```python
from build123d import *

# Parameters (mm, degrees)
SKETCH1_W           = 37
SKETCH1_H           = 22.3
BOSS_EXTRUDE1_DEPTH = 19.13
BOSS_EXTRUDE2_DEPTH = 22.3


with BuildPart() as part:
    # Sketch1 → Boss-Extrude1 (new body)
    with BuildSketch(Plane(origin=(0, 0, 0), x_dir=(1, 0, 0), z_dir=(0, 1, 0))):
        Rectangle(SKETCH1_W, SKETCH1_H)
    extrude(amount=BOSS_EXTRUDE1_DEPTH)

    # Sketch2 → Boss-Extrude2 (add)
    with BuildSketch(Plane.XY.offset(11.15)):
        with BuildLine():
            Line((4e-09, 0), (-18.5, 0))
            Line((-18.5, 0), (-18.5, -18.5))
            ThreePointArc((-18.5, -18.5), (-13.081475451, -5.418524547), (4e-09, 0))
        make_face()
        with BuildLine():
            Line((18.5, 0), (4e-09, 0))
            ThreePointArc((4e-09, 0), (13.081475453, -5.418524549), (18.5, -18.5))
            Line((18.5, -18.5), (18.5, 0))
        make_face()
    extrude(amount=-BOSS_EXTRUDE2_DEPTH)


solid = part.part
```
Verification items for the finished model (mm, model axes). Round coordinates to 2 decimals unless told otherwise and drop trailing zeros. Order: outer loops, then holes, each group sorted by start corner. A loop starts at its lowest first (then second) coordinate and runs counter-clockwise, first axis right, second up. Notation, with made-up numbers: (-29.75, -6) -> (15.25, -6) arc R27 cw to (15.25, 23) -> close; hole circle Ø3 at (36.5, 40.25). An arc over 180 degrees is marked (long way). Put each result on its own line as item: value. Start each with the question number.
(1) Section check A-A (y = -9). Enter the section's corners in (x, z), then the cut area to 3 significant figures.
(2) Depth check by flat-ended pin: pin 1 Ø3 at (x, z) = (-9, 4) entering from -Y; pin 2 Ø10 at (x, y) = (5.5, -8.5) entering from -Z. Enter the tip coordinate at first touch or a pass-through.
(3) Material ranges on line 1 along X through (y, z) = (-15, 0); line 2 along X through (y, z) = (-4, 0); line 3 along Y through (x, z) = (-2.5, 0), recorded low to high.
(4) Section check B-B (z = -7.25). Enter the section's corners in (x, y).
(5) Section check C-C (x = 6). Enter the section's corners in (y, z).
Completed:
1. outline: (-18.5, -11.15) -> (-15.87, -11.15) -> (-15.87, 11.15) -> (-18.5, 11.15) -> close; (15.87, -11.15) -> (18.5, -11.15) -> (18.5, 11.15) -> (15.87, 11.15) -> close
1. area: 117 mm2
2. pin 1: stops at y = -3.27
2. pin 2: passes through
3. line 1: x = -18.5 to -18.17, 18.17 to 18.5
3. line 2: x = -18.5 to -11.49, 11.49 to 18.5
3. line 3: y = -0.17 to 19.13
4. outline: (-18.5, -18.5) arc R18.5 cw to (18.5, -18.5) -> (18.5, 19.13) -> (-18.5, 19.13) -> close
5. outline: (-1, -11.15) -> (19.13, -11.15) -> (19.13, 11.15) -> (-1, 11.15) -> close
